from build123d import *

# Parameters (mm, degrees)
BOSS_EXTRUDE1_DEPTH                 = 38.1
SKETCH2_W                           = 41.275
SKETCH2_H                           = 44.704
END_CAPS_DEPTH                      = 6.35
CHANNEL_COUNTERSINK_PRE_D           = 8.4328
CHANNEL_COUNTERSINK_PRE_DEPTH       = 9.525
CHANNEL_COUNTERSINK_PRE_CSINK_D     = 16.129
CHANNEL_COUNTERSINK_PRE_CSINK_ANGLE = 100
CHANNEL_COUNTERSINK_PRE_TIP         = 2.533468714
MOUNTING_COUNTERSINK_D              = 8.4328
MOUNTING_COUNTERSINK_CSINK_D        = 16.129
MOUNTING_COUNTERSINK_CSINK_ANGLE    = 100
SKETCH13_W                          = 16.129
SKETCH13_H                          = 4.7625
CHANNEL_TOP_AND_BOTTOM_DEPTH        = 51.8
CHANNEL_COUNTERSINK_D               = 8.4328
CHANNEL_COUNTERSINK_DEPTH           = 4.7625
CHANNEL_COUNTERSINK_CSINK_D         = 16.129
CHANNEL_COUNTERSINK_CSINK_ANGLE     = 100
CHANNEL_COUNTERSINK_TIP             = 2.533468714
SKETCH16_W                          = 16.129
SKETCH16_H                          = 3.175
CHANNEL_LEFT_RIGHT_DEPTH            = 45.704
SKETCH17_W                          = 16.129
SKETCH17_H                          = 6.477
CUT_EXTRUDE3_DEPTH                  = 51.8
F_5_16_0_47_DIAMETER_HOLE1_D        = 11.938
F_5_16_0_47_DIAMETER_HOLE1_DEPTH    = 14.859


with BuildPart() as part:
    # Sketch1 → Boss-Extrude1 (new body)
    with BuildSketch(Plane(origin=(0, 0, 0), x_dir=(1, 0, 0), z_dir=(0, 1, 0))):
        Polygon((0, 0), (-41.275, 0), (-41.275, -14.859), (-9.525, -14.859), (-9.525, -35.179), (-41.275, -35.179), (-41.275, -44.704), (0, -44.704), align=None)
    extrude(amount=BOSS_EXTRUDE1_DEPTH)

    # Sketch2 → End Caps (add)
    with BuildSketch(Plane(origin=(0, 38.1, 0), x_dir=(-1, 0, 0), z_dir=(0, 1, 0))):
        with Locations((20.6375, 22.352)):
            Rectangle(SKETCH2_W, SKETCH2_H)
    end_caps = extrude(amount=END_CAPS_DEPTH)

    # Mirror1: End Caps across plane
    add(end_caps.mirror(Plane(origin=(0, 19.05, 0), x_dir=(0, 0, 1), z_dir=(0, -1, 0))))

    # Channel Countersink-PRE
    with Locations(Plane.XY.offset(44.704)):
        with Locations((-31.115, 19.05)):
            CounterSinkHole(CHANNEL_COUNTERSINK_PRE_D / 2, CHANNEL_COUNTERSINK_PRE_CSINK_D / 2, depth=CHANNEL_COUNTERSINK_PRE_DEPTH, counter_sink_angle=CHANNEL_COUNTERSINK_PRE_CSINK_ANGLE)
            with Locations((0, 0, -(CHANNEL_COUNTERSINK_PRE_DEPTH + CHANNEL_COUNTERSINK_PRE_TIP / 2))):  # 118° drill point
                Cone(0, CHANNEL_COUNTERSINK_PRE_D / 2, CHANNEL_COUNTERSINK_PRE_TIP, mode=Mode.SUBTRACT)

    # Mounting Countersink (through all)
    with Locations(Plane.ZY.offset(9.525)):
        with Locations((25.019, 19.05)):
            CounterSinkHole(MOUNTING_COUNTERSINK_D / 2, MOUNTING_COUNTERSINK_CSINK_D / 2, counter_sink_angle=MOUNTING_COUNTERSINK_CSINK_ANGLE)

    # Sketch13 → Channel Top and Bottom (cut, through all)
    with BuildSketch(Plane.XZ.offset(6.35)):
        with Locations((-31.115, 42.32275)):
            Rectangle(SKETCH13_W, SKETCH13_H)
    extrude(amount=-CHANNEL_TOP_AND_BOTTOM_DEPTH, mode=Mode.SUBTRACT)

    # Channel Countersink
    with Locations(Plane.XY.offset(39.9415)):
        with Locations((-31.115, 19.05)):
            CounterSinkHole(CHANNEL_COUNTERSINK_D / 2, CHANNEL_COUNTERSINK_CSINK_D / 2, depth=CHANNEL_COUNTERSINK_DEPTH, counter_sink_angle=CHANNEL_COUNTERSINK_CSINK_ANGLE)
            with Locations((0, 0, -(CHANNEL_COUNTERSINK_DEPTH + CHANNEL_COUNTERSINK_TIP / 2))):  # 118° drill point
                Cone(0, CHANNEL_COUNTERSINK_D / 2, CHANNEL_COUNTERSINK_TIP, mode=Mode.SUBTRACT)

    # Sketch16 → Channel Left Right (cut, through all)
    with BuildSketch(Plane(origin=(0, 0, 0), x_dir=(1, 0, 0), z_dir=(0, 0, -1))):
        with Locations((-31.115, 4.7625)):
            Rectangle(SKETCH16_W, SKETCH16_H)
    channel_left_right = extrude(amount=-CHANNEL_LEFT_RIGHT_DEPTH, mode=Mode.SUBTRACT)

    # Sketch17 → Cut-Extrude3 (cut, through all)
    with BuildSketch(Plane(origin=(0, 44.45, 0), x_dir=(-1, 0, 0), z_dir=(0, 1, 0))):
        with Locations((31.115, 3.2385)):
            Rectangle(SKETCH17_W, SKETCH17_H)
    extrude(amount=-CUT_EXTRUDE3_DEPTH, mode=Mode.SUBTRACT)

    # Mirror3: Channel Left Right across plane
    add(channel_left_right.mirror(Plane(origin=(0, 19.05, 0), x_dir=(0, 0, 1), z_dir=(0, -1, 0))), mode=Mode.SUBTRACT)

    # 5/16 (0.47) Diameter Hole1
    with Locations(Plane(origin=(0, 0, 0), x_dir=(1, 0, 0), z_dir=(0, 0, -1))):
        with Locations((-31.115, -19.05)):
            Hole(F_5_16_0_47_DIAMETER_HOLE1_D / 2, depth=F_5_16_0_47_DIAMETER_HOLE1_DEPTH)


solid = part.part
CAD build for the part. Positions are in the model's coordinates, mm. A direction names the side the tool comes from. Round coordinates to 2 decimals unless told otherwise and drop trailing zeros. Order: outer loops, then holes, each group sorted by start corner. A loop starts at its lowest first (then second) coordinate and runs counter-clockwise, first axis right, second up. Notation, with made-up numbers: (-5.75, -34) - (44.25, -34) arc R33 cw to (44.25, 1) - close; hole circle Ø11 at (76.5, -26.75). An arc over 180 degrees is marked (long way). Return JSON: item names as keys, results as strings.
(1) Pin check, flat tips, straight feed: pin 1 Ø10 at (x, z) = (-30, 26.5) entering from +Y (3 decimals); pin 2 Ø13.5 at (y, z) = (19.05, 25.019) entering from -X; pin 3 Ø9.5 at (x, y) = (-31.115, 19.05) entering from -Z. Stop position of each tip, or through.
Answer key:
{"pin 1": "stops at y = 41.275", "pin 2": "stops at x = -8.42", "pin 3": "stops at z = 35.18"}
(2) Cut at B-B (y = -1). Give the cut face in (x, z) (1 decimal), then the cut area to 3 significant figures.
Answer key:
{"outline": "(-41.3, 0) - (-39.2, 0) - (-39.2, 6.5) - (-23.1, 6.5) - (-23.1, 0) - (0, 0) - (0, 44.7) - (-23.1, 44.7) - (-23.1, 39.9) - (-39.2, 39.9) - (-39.2, 44.7) - (-41.3, 44.7) - close", "area": "1,660 mm^2"}
(3) Tool access for faces 1 (the face through (-23.05, 17, 6)), 2 (the face through (-31, 41.275, 23)), 3 (the face through (-25, 38.1, 25)), 4 (the face through (-31, -3.175, 23)): list every direction of +Z, -Z, +X, -X, +Y, -Y with a clear straight run to the whole face (end or side of a thin tool).
Answer key:
{"face 1": "none", "face 2": "+Z, -Z, +Y", "face 3": "-X", "face 4": "+Z, -Z, -Y"}
(4) Cut at C-C (x = -2.5). Give the cut face in (y, z), then the cut area to 3 significant figures.
Answer key:
{"outline": "(-6.35, 0) - (44.45, 0) - (44.45, 44.7) - (-6.35, 44.7) - close; hole circle Ø8.43 at (19.05, 25.02)", "area": "2,220 mm^2"}
(5) Wall check: probe 1 along Z at (x, y) = (-20.5, 23); probe 2 along X at (y, z) = (-3.5, 10) (1 decimal); probe 3 along Z at (x, y) = (-25.5, 7). Give the ranges that are in metal, low to high. Write a range as from..to.
Answer key:
{"probe 1": "z = 0..14.86, 35.18..44.7", "probe 2": "x = -41.3..-39.2, -23.1..0", "probe 3": "z = 6.48..14.86, 35.18..39.94"}
(6) Pull direction X, two halves, no side cores. Call faces 5 (the face through (0, 19, 17)), 6 (the face through (-11, 19, 44.704)), 7 (the face through (-34.3, 14, 10.7)): +X half, -X half, draft (parallel to the pull), parting line (faces both ways), or undercut.
Answer key:
{"face 5": "+X half", "face 6": "draft", "face 7": "undercut"}
